from build123d import *

# Parameters (mm, degrees)
F0_R      = 6.25
F1_DEPTH  = 13.5
F2_R      = 12
F2_R_2    = 1.5
F2_R_3    = 6.25
F3_DEPTH  = 1
F4_R      = 5.5
F4_R_2    = 2.5
F5_DEPTH  = 1
F6_DEPTH  = 3
F7_R      = 3
F7_R_2    = 2.5
F8_DEPTH  = 1
F9_R      = 5.25
F10_DEPTH = 1.5
F11_R     = 0.5
F12_DEPTH = 5
F13_R     = 0.5
F14_DEPTH = 5


with BuildPart() as f1:
    # F0 (on Front) → F1 (new body)
    with BuildSketch(Plane.XZ):
        Circle(F0_R)
    extrude(amount=F1_DEPTH)

    # F2 (on face) → F3 (join)
    with BuildSketch(Plane(origin=(0, 0, 0), x_dir=(-1, 0, 0), z_dir=(0, 1, 0))):
        Circle(F2_R)
        with Locations((-7.7942286341, -4.5)):
            Circle(F2_R_2, mode=Mode.SUBTRACT)
        with Locations((7.7942286341, -4.5)):
            Circle(F2_R_2, mode=Mode.SUBTRACT)
        Circle(F2_R_3, mode=Mode.SUBTRACT)
        with Locations((0, 9)):
            Circle(F2_R_2, mode=Mode.SUBTRACT)
        Circle(F2_R_3)
    extrude(amount=F3_DEPTH)

    # F4 (on face) → F5 (join)
    with BuildSketch(Plane(origin=(0, 1, 0), x_dir=(-1, 0, 0), z_dir=(0, 1, 0))):
        Circle(F4_R)
        Circle(F4_R_2, mode=Mode.SUBTRACT)
    extrude(amount=F5_DEPTH)

    # F6 (add): a face of the model
    f6_faces = [f1.faces().sort_by_distance(p)[0] for p in [
        (0, 1, 0),
    ]]
    extrude(f6_faces, amount=F6_DEPTH)

    # F7 (on face) → F8 (cut)
    with BuildSketch(Plane(origin=(0, 2, 0), x_dir=(-1, 0, 0), z_dir=(0, 1, 0))):
        Circle(F7_R)
        Circle(F7_R_2, mode=Mode.SUBTRACT)
    extrude(amount=-F8_DEPTH, mode=Mode.SUBTRACT)

    # F9 (on face) → F10 (cut)
    with BuildSketch(Plane.XZ.offset(13.5)):
        Circle(F9_R)
    extrude(amount=-F10_DEPTH, mode=Mode.SUBTRACT)

    # F11 (on face) → F12 (join)
    with BuildSketch(Plane.XZ.offset(12)):
        with Locations((-4.3, -1.1)):
            Circle(F11_R)
        with Locations((-4.3, 0)):
            Circle(F11_R)
        with Locations((-4.3, 1.1)):
            Circle(F11_R)
        with Locations((4.3, 1.1)):
            Circle(F11_R)
        with Locations((4.3, 0)):
            Circle(F11_R)
        with Locations((4.3, -1.1)):
            Circle(F11_R)
    extrude(amount=F12_DEPTH)

    # F13 (on face) → F14 (join)
    with BuildSketch(Plane(origin=(0, 4, 0), x_dir=(-1, 0, 0), z_dir=(0, 1, 0))):
        with Locations((-0.875, -1.5155444566)):
            Circle(F13_R)
        with Locations((0.875, -1.5155444566)):
            Circle(F13_R)
        with Locations((1.75, 0)):
            Circle(F13_R)
        with Locations((0.875, 1.5155444566)):
            Circle(F13_R)
        with Locations((-0.875, 1.5155444566)):
            Circle(F13_R)
        with Locations((-1.75, 0)):
            Circle(F13_R)
    extrude(amount=F14_DEPTH)


solid = f1.part
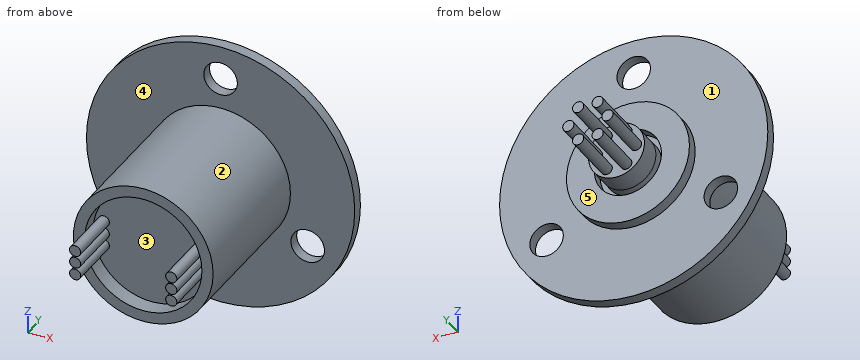
Input: part model. Units: mm. Frame: model coordinates. Face numbers are marked on the shaded views. A direction names the side the tool comes from. Coordinates: 2 decimals unless noted, no trailing zeros. Loops run counter-clockwise (first coordinate to the right, second up) from the corner with the lowest first, then second, coordinate; pieces in that order, holes last.
(1) Section D-D on z = 9. Return the cut outline in (x, y), then the cut area to 3 significant figures.
(2) Pull-direction query (X, two-part tool) for the marked faces 1, 2 and 3; classes: released by +X, released by -X, zero draft, split by the parting line, or undercut.
(3) Section B-B on z = -4.5. Return the cut outline in (x, y), then the cut area to 3 significant figures.
(4) Section A-A on x = 0. Return the cut outline in (y, z).
(5) Section C-C on y = 7.25. Return the cut outline in (x, z) (3 decimals), then the cut area to 3 significant figures.
(6) First-contact query: pin 1 Ø4 at (x, z) = (2, 3) entering from -Y; pin 2 Ø1.5 at (x, y) = (-1.5, -3.5) entering from +Z; pin 3 Ø12 at (y, z) = (0, 6.5) entering from +X. Flat tips, straight axial feed; report the tip coordinate or a pass-through.
(7) Material intervals for probe 1 along Z at (x, y) = (0, 0.8); probe 2 along Y at (x, z) = (-3.75, -10); probe 3 along Z at (x, y) = (0, -12.55), sorted ascending.
(8) Set-up query: the marked faces 4 and 5. Return all of +Z, -Z, +X, -X, +Y, -Y with unobstructed straight access to the full face (end or side cutting, diameter ignored); none if empty.
Data:
1. outline: (-7.94, 0) - (-1.5, 0) - (-1.5, 1) - (-7.94, 1) - close; (1.5, 0) - (7.94, 0) - (7.94, 1) - (1.5, 1) - close
1. area: 12.9 mm2
2. face 1: zero draft
2. face 2: split by the parting line
2. face 3: undercut
3. outline: (-11.12, 0) - (-9.29, 0) - (-9.29, 1) - (-11.12, 1) - close; (-6.29, 0) - (-4.34, 0) - (-4.34, -13.5) - (-2.7, -13.5) - (-2.7, -12) - (2.7, -12) - (2.7, -13.5) - (4.34, -13.5) - (4.34, 0) - (6.29, 0) - (6.29, 1) - (3.16, 1) - (3.16, 2) - (-3.16, 2) - (-3.16, 1) - (-6.29, 1) - close; (9.29, 0) - (11.12, 0) - (11.12, 1) - (9.29, 1) - close
3. area: 132 mm2
4. outline: (-13.5, -6.25) - (0, -6.25) - (0, -12) - (1, -12) - (1, -5.5) - (2, -5.5) - (2, -3) - (1, -3) - (1, -2.5) - (4, -2.5) - (4, 2.5) - (1, 2.5) - (1, 3) - (2, 3) - (2, 5.5) - (1, 5.5) - (1, 7.5) - (0, 7.5) - (0, 6.25) - (-13.5, 6.25) - (-13.5, 5.25) - (-12, 5.25) - (-12, -5.25) - (-13.5, -5.25) - close; (0, 10.5) - (1, 10.5) - (1, 12) - (0, 12) - close
5. outline: circle Ø1 at (-1.75, 0); circle Ø1 at (-0.875, -1.516); circle Ø1 at (-0.875, 1.516); circle Ø1 at (0.875, -1.516); circle Ø1 at (0.875, 1.516); circle Ø1 at (1.75, 0)
5. area: 4.71 mm2
6. pin 1: stops at y = -13.5
6. pin 2: stops at z = 6.2
6. pin 3: stops at x = 11.99
7. probe 1: z = -12 to 7.5, 10.5 to 12
7. probe 2: y = 0 to 1
7. probe 3: z = -6.25 to -5.25, 5.25 to 6.25
8. face 4: -Y
8. face 5: +Y
